Here's how the part is built. I have some questions about the finished solid (model axes, mm). A direction names the side the tool comes from. Round coordinates to 2 decimals unless told otherwise and drop trailing zeros. Loops run counter-clockwise (first coordinate to the right, second up) from the corner with the lowest first, then second, coordinate; pieces in that order, holes last. Notation, with made-up numbers: M 7,89 L 43,89 A26 ccw 43,108 Z; hole C -26.5,89.5 d9. An arc over 180 degrees is marked long. Write each question's results on one line, items separated by ' | '. Start each with the question number.
```python
from build123d import *

# Parameters (mm, degrees)
F2_DEPTH = 50
F3_DEPTH = 25
F4_DEPTH = 25
F6_DEPTH = 75
F7_R     = 2


# Not quite as in the source:
# - the program builds the solid bodies; features that only make, move or delete a surface that nothing else refers to are left out


with BuildPart() as f2:
    # F0 (on Front) → F2 (new body, symmetric)
    with BuildSketch(Plane.XZ):
        with BuildLine():
            ThreePointArc((86.0395411487, 78.1614595205), (84.6450154703, 80.8109382584), (82.8911252312, 83.2375219638))
            Line((82.8911252312, 83.2375219638), (82.8911252312, 69.6372875124))
            Line((82.8911252312, 69.6372875124), (98.3350202441, 69.6372875124))
            Line((98.3350202441, 69.6372875124), (98.3350202441, 78.1614595205))
            Line((98.3350202441, 78.1614595205), (86.0395411487, 78.1614595205))
        make_face()
        with BuildLine():
            Line((141.6950114063, 90.9081755561), (82.8911252312, 90.9081755561))
            Line((82.8911252312, 90.9081755561), (82.8911252312, 83.2375219638))
            ThreePointArc((82.8911252312, 83.2375219638), (84.6450154703, 80.8109382584), (86.0395411487, 78.1614595205))
            Line((86.0395411487, 78.1614595205), (98.3350202441, 78.1614595205))
            Line((98.3350202441, 78.1614595205), (98.3350202441, 69.6372875124))
            Line((98.3350202441, 69.6372875124), (82.8911252312, 69.6372875124))
            Line((82.8911252312, 69.6372875124), (82.8911252312, 50.8714897913))
            Line((82.8911252312, 50.8714897913), (141.6950114063, 50.8714897913))
            Line((141.6950114063, 50.8714897913), (141.6950114063, 90.9081755561))
        make_face()
        with BuildLine():
            Line((45.431509614, 69.6372875124), (45.431509614, 12))
            Line((45.431509614, 12), (53.955681622, 12))
            Line((53.955681622, 12), (53.955681622, 69.6372875124))
            ThreePointArc((53.955681622, 69.6372875124), (66.6301945598, 82.3118004502), (79.3047074976, 69.6372875124))
            Line((79.3047074976, 69.6372875124), (82.8911252312, 69.6372875124))
            Line((82.8911252312, 69.6372875124), (82.8911252312, 83.2375219638))
            ThreePointArc((82.8911252312, 83.2375219638), (59.3957665519, 89.563333152), (45.431509614, 69.6372875124))
        make_face()
    extrude(amount=F2_DEPTH, both=True)

    # F0 (on Front) → F3 (join)
    with BuildSketch(Plane.XZ):
        with BuildLine():
            add(Edge.make_bspline(
                [(-53.955681622, 12), (-55.4214757867, 72.6385811269), (29.6854469925, 93.0915244818), (82.8911252312, 90.9081755561)],
                knots=[0, 0, 0, 0, 157.9669228526, 157.9669228526, 157.9669228526, 157.9669228526], degree=3))
            Line((-53.955681622, 12), (45.431509614, 12))
            Line((45.431509614, 12), (45.431509614, 69.6372875124))
            ThreePointArc((45.431509614, 69.6372875124), (59.3957665519, 89.563333152), (82.8911252312, 83.2375219638))
            Line((82.8911252312, 83.2375219638), (82.8911252312, 90.9081755561))
        make_face()
        Polygon((45.431509614, 12), (-53.955681622, 12), (-53.955681622, -12), (53.955681622, -12), (53.955681622, 12), align=None)
        with BuildLine():
            Line((45.431509614, 69.6372875124), (45.431509614, 12))
            Line((45.431509614, 12), (53.955681622, 12))
            Line((53.955681622, 12), (53.955681622, 69.6372875124))
            ThreePointArc((53.955681622, 69.6372875124), (66.6301945598, 82.3118004502), (79.3047074976, 69.6372875124))
            Line((79.3047074976, 69.6372875124), (82.8911252312, 69.6372875124))
            Line((82.8911252312, 69.6372875124), (82.8911252312, 83.2375219638))
            ThreePointArc((82.8911252312, 83.2375219638), (59.3957665519, 89.563333152), (45.431509614, 69.6372875124))
        make_face()
        with BuildLine():
            Line((141.6950114063, 90.9081755561), (82.8911252312, 90.9081755561))
            Line((82.8911252312, 90.9081755561), (82.8911252312, 83.2375219638))
            ThreePointArc((82.8911252312, 83.2375219638), (84.6450154703, 80.8109382584), (86.0395411487, 78.1614595205))
            Line((86.0395411487, 78.1614595205), (98.3350202441, 78.1614595205))
            Line((98.3350202441, 78.1614595205), (98.3350202441, 69.6372875124))
            Line((98.3350202441, 69.6372875124), (82.8911252312, 69.6372875124))
            Line((82.8911252312, 69.6372875124), (82.8911252312, 50.8714897913))
            Line((82.8911252312, 50.8714897913), (141.6950114063, 50.8714897913))
            Line((141.6950114063, 50.8714897913), (141.6950114063, 90.9081755561))
        make_face()
        with BuildLine():
            ThreePointArc((86.0395411487, 78.1614595205), (84.6450154703, 80.8109382584), (82.8911252312, 83.2375219638))
            Line((82.8911252312, 83.2375219638), (82.8911252312, 69.6372875124))
            Line((82.8911252312, 69.6372875124), (98.3350202441, 69.6372875124))
            Line((98.3350202441, 69.6372875124), (98.3350202441, 78.1614595205))
            Line((98.3350202441, 78.1614595205), (86.0395411487, 78.1614595205))
        make_face()
    extrude(amount=F3_DEPTH)

    # F0 (on Front) → F4 (join, symmetric)
    with BuildSketch(Plane.XZ):
        Polygon((45.431509614, 12), (-53.955681622, 12), (-53.955681622, -12), (53.955681622, -12), (53.955681622, 12), align=None)
    extrude(amount=F4_DEPTH, both=True)

    # F1 (on face) → F6 (join, symmetric)
    with BuildSketch(Plane.XZ):
        Polygon((53.955681622, 12), (45.431509614, 12), (-53.955681622, 12), (-53.955681622, -12), (53.955681622, -12), align=None)
    extrude(amount=F6_DEPTH, both=True)

    # F7
    f7_edges = [f2.edges().sort_by_distance(p)[0] for p in [
        (53.955682, -75, 0),
        (0, -75, 12),
        (-53.955682, -75, 0),
        (0, -75, -12),
        (53.955682, 75, 0),
        (0, 75, 12),
        (-53.955682, 75, 0),
        (0, 75, -12),
    ]]
    fillet(f7_edges, radius=F7_R)


solid = f2.part
```
1. I need wall thicknesses on line 1 along X through (y, z) = (-25.5, 61); line 2 along Z through (x, y) = (12, -42); line 3 along Y through (x, z) = (-30.5, 42). Which ranges of each line are inside material? Lowest first, please.
2. For pin 1 (20 mm diameter, centred on y = -36.5, z = 28, fed in from -X); pin 2 (2.5 mm diameter, centred on y = 29, z = 85.5, fed in from -X); pin 3 (5 mm diameter, centred on x = 34, z = 60, fed in from +Y), each with a flat end and sliding along its axis, tell me the tip position at first contact or that it passes through.
3. Which directions (+Z, -Z, +X, -X, +Y, -Y) give clear straight access to the entire face, cutting with the end or side of a thin tool? Please do faces 4 (the face through (82.891, 1, 60)), 5 (the face through (93, -50, 70)), 6 (the face through (45.432, -38, 41)).
4. I want a section at A-A on y = 45. List the corners of the cut face in (x, z) for me, plus the area to 3 significant figures.
5. I want a section at B-B on y = -58.5. List the corners of the cut face in (x, z) for me, plus the area to 3 significant figures.
6. If we mould it in two halves opening along X, with no side actions, what happens to faces 1 (the face through (53.956, -1, 28)), 2 (the face through (45.432, 25, 41)), 3 (the face through (1, -49, 12))? For each: released by +X, released by -X, zero draft, split by the parting line, or undercut.
Outcome:
1) line 1: 45.43 to 53.96, 82.89 to 141.7 | line 2: -12 to 12 | line 3: -25 to 0
2) pin 1: x = 45.43 | pin 2: x = 51.27 | pin 3: y = 0
3) face 4: -Z, +Y, -Y | face 5: +Z, +X, -X, -Y | face 6: +Z, -X, -Y
4) outline: M -53.96,-12 L 53.96,-12 L 53.96,69.64 A12.67 cw 79.3,69.64 L 82.89,69.64 L 82.89,50.87 L 141.7,50.87 L 141.7,90.91 L 82.89,90.91 L 82.89,83.24 A21.2 ccw 45.43,69.64 L 45.43,12 L -53.96,12 Z | area: 5,840 mm2
5) outline: M -53.96,-12 L 53.96,-12 L 53.96,12 L -53.96,12 Z | area: 2,590 mm2
6) face 1: undercut | face 2: released by -X | face 3: zero draft
